For this review, take the finished solid that the model builds, in its own axes (mm). Face numbers are marked on the shaded views. A direction names the side the tool comes from. Give positions to 0.01 mm unless a question says otherwise; leave off trailing zeros. Write each loop counter-clockwise with the first axis right and the second up, starting at its lowest first coordinate (ties: lowest second). Pieces come first, ordered by that corner, then holes. Notation, with made-up numbers: M 13,50 L 17,50 A26 ccw 17,78 Z; hole C -15,65 d2. An arc over 180 degrees is marked long. Answer as a JSON object with one key per item and string values. Group by question number.
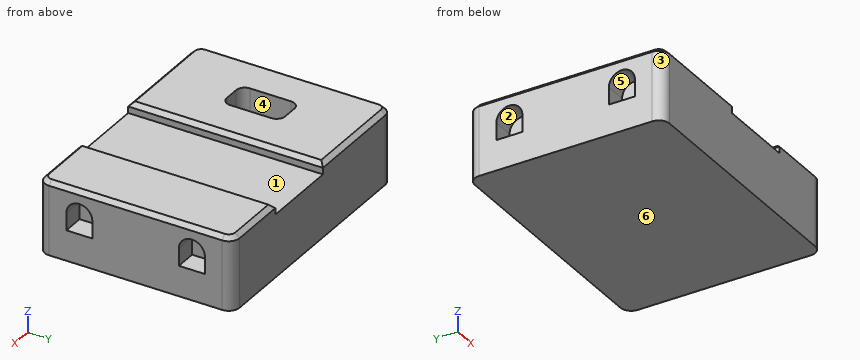
Solid Edge part; units mm, degrees
sketch "Sketch1" plane through (0, 0, 0) normal (0, 0, 1) x (1, 0, 0)
  line L0 (-30, -22.5) -> (30, -22.5)
  line L1 (30, -22.5) -> (30, 22.5)
  line L2 (30, 22.5) -> (-30, 22.5)
  line L3 (-30, 22.5) -> (-30, -22.5)
  dimension "D1" = 30
  dimension "D2" = 30
extrude "Protrusion1" add sketch "Sketch1" along normal blind 17
fillet "Verrundung_1" radius 2.5 4 edges at (-30, 22.5, 8.5) (30, 22.5, 8.5) (30, -22.5, 8.5) (-30, -22.5, 8.5)
chamfer "Fase_1" distance 1 angle 45 7 edges at (30, 0, 17) (0, 22.5, 17) (-29.2678, 21.7678, 17) (-30, 0, 17) (-29.2678, -21.7678, 17) (0, -22.5, 17) (29.2678, -21.7678, 17)
sketch "Sketch2" plane through (-30, 0, 4.75) normal (-1, 0, 0) x (0, 0, 1)
  line L0 (6.25, 16) -> (2.25, 16)
  line L1 (2.25, 16) -> (2.25, 10)
  line L2 (6.25, 10) -> (2.25, 10)
  arc A0 (6.25, 10) -> (6.25, 16) centre (6.25, 13) ccw
extrude "ExtrudedCutout_5" cut sketch "Sketch2" against normal blind 5
mirror "Mirror1" about plane through (0, 0, 0) normal (0, -1, 0) of "ExtrudedCutout_5"
mirror "Mirror2" about plane through (0, 0, 0) normal (1, 0, 0) of "Mirror1", "ExtrudedCutout_5"
sketch "Sketch3" plane through (0, -22.5, 4.75) normal (0, -1, 0) x (1, 0, 0)
  line L0 (-4, 12.25) -> (-4, 9.75)
  line L1 (-4, 9.75) -> (14, 9.75)
  line L2 (14, 9.75) -> (14, 12.25)
  dimension "D1" = 4
extrude "ExtrudedCutout_7" cut sketch "Sketch3" against normal blind 55.5038 material side at (-3.95, -22.5, 15.75)
chamfer "Chamfer_3" distance 1 angle 45 2 edges at (14, 0, 17) (-4, 0, 17)
sketch "Sketch4" plane through (-17, 0, 17) normal (0, 0, 1) x (1, 0, 0)
  line L0 (-4, -6.75) -> (3.5, -6.75)
  line L1 (3.5, -6.75) -> (3.5, 6.75)
  line L2 (3.5, 6.75) -> (-4, 6.75)
  line L3 (-4, 6.75) -> (-4, -6.75)
  dimension "D1" = 3.5
  dimension "D2" = 3.5
extrude "ExtrudedCutout_8" cut sketch "Sketch4" against normal blind 10
fillet "Round_3" radius 2 4 edges at (-21, 6.75, 12) (-13.5, 6.75, 12) (-13.5, -6.75, 12) (-21, -6.75, 12)
Item 1: Consider section B-B (y = -13). Give the boundary of the cut face in (x, z), plus the area to 3 significant figures.
Item 2: Insertion check: P1, Ø4, axis at x = -16.5, y = 0, coming from the +Z side. The pin has a flat end and moves straight along its axis. Give the tip position at first contact, or say it passes through.
Item 3: Consider section D-D (y = 19). Give the boundary of the cut face in (x, z).
Item 4: Consider section C-C (x = 4.5). Give the boundary of the cut face in (y, z), plus the area to 4 significant figures.
Item 5: To check wall thickness, follow probe 1 along X at (y, z) = (5, 15.25); probe 2 along X at (y, z) = (3.5, 12); probe 3 along X at (y, z) = (15.5, 16). State the ranges of each line that lie inside material, in increasing order.
Item 6: Machinability: for the marked faces 4, 5 and 6, which of the approach directions +Z, -Z, +X, -X, +Y, -Y give a long, thin tool a straight path to every point of the face, cutting with its end or side? Answer none if there is none.
Item 7: Draft analysis for pull direction X (two halves, no side actions). For the marked faces 1, 2 and 3, state which applies: released by +X, released by -X, zero draft, split by the parting line, or undercut.
Result set:
{
 "1": {"outline": "M -30,0 L 30,0 L 30,7 L 25,7 L 25,14 L 30,14 L 30,16 L 29,17 L 15,17 L 14,16 L 14,14.5 L -4,14.5 L -4,16 L -5,17 L -29,17 L -30,16 L -30,14 L -25,14 L -25,7 L -30,7 Z", "area": "903 mm^2"},
 "2": {"P1": "stops at z = 7"},
 "3": {"outline": "M -30,0 L 30,0 L 30,16 L 29,17 L 15,17 L 14,16 L 14,14.5 L -4,14.5 L -4,16 L -5,17 L -29,17 L -30,16 Z"},
 "4": {"outline": "M -22.5,0 L 22.5,0 L 22.5,14.5 L -22.5,14.5 Z", "area": "652.5 mm^2"},
 "5": {"probe 1": "x = -30 to -20.98, -13.52 to -4, 14 to 30", "probe 2": "x = -30 to -21, -13.5 to 30", "probe 3": "x = -30 to -4, 14 to 30"},
 "6": {"face 4": "+Z", "face 5": "-X", "face 6": "-Z, +X, -X, +Y, -Y"},
 "7": {"face 1": "undercut", "face 2": "zero draft", "face 3": "released by -X"}
}
